from build123d import *

# Parameters (mm, degrees)
BOSS_EXTRUDE1_DEPTH = 1.905
SKETCH2_R           = 3.4925
SKETCH2_R_2         = 2.54
BOSS_EXTRUDE2_DEPTH = 50.8
FILLET2_R           = 0.635
SCALE1_SCALE        = 1.5


with BuildPart() as part:
    # Sketch1 → Boss-Extrude1 (new body)
    with BuildSketch(Plane(origin=(0, 0, 0), x_dir=(1, 0, 0), z_dir=(0, 1, 0))):
        with BuildLine():
            Line((-6.0325, -4.7625), (-6.0325, 4.7625))
            ThreePointArc((-6.0325, 4.7625), (-5.660525612, 5.660525612), (-4.7625, 6.0325))
            Line((-4.7625, 6.0325), (4.7625, 6.0325))
            ThreePointArc((4.7625, 6.0325), (5.660525612, 5.660525612), (6.0325, 4.7625))
            Line((6.0325, 4.7625), (6.0325, -4.7625))
            ThreePointArc((6.0325, -4.7625), (5.660525612, -5.660525612), (4.7625, -6.0325))
            Line((4.7625, -6.0325), (-4.7625, -6.0325))
            ThreePointArc((-4.7625, -6.0325), (-5.660525612, -5.660525612), (-6.0325, -4.7625))
        make_face()
    extrude(amount=BOSS_EXTRUDE1_DEPTH)

    # Sketch2 → Boss-Extrude2 (add)
    with BuildSketch(Plane.XZ):
        with Locations(Location((0, 0, 0), (0, 0, 270))):
            Circle(SKETCH2_R)
        with Locations(Location((0, 0, 0), (0, 0, 270))):
            Circle(SKETCH2_R_2, mode=Mode.SUBTRACT)
    extrude(amount=BOSS_EXTRUDE2_DEPTH)

    # Fillet2
    fillet2_edges = [part.edges().sort_by_distance(p)[0] for p in [
        (-5.660525612, 1.905, -5.660525612),
        (0, 0, -6.0325),
        (5.660525612, 0, -5.660525612),
        (-6.0325, 1.905, 0),
        (-5.660525612, 1.905, 5.660525612),
        (0, 1.905, 6.0325),
        (5.660525612, 1.905, 5.660525612),
        (6.0325, 1.905, 0),
        (5.660525612, 1.905, -5.660525612),
        (0, 1.905, -6.0325),
        (6.0325, 0, 0),
        (5.660525612, 0, 5.660525612),
        (0, 0, 6.0325),
        (-5.660525612, 0, 5.660525612),
        (-6.0325, 0, 0),
        (-5.660525612, 0, -5.660525612),
    ]]
    fillet(fillet2_edges, radius=FILLET2_R)


with BuildPart() as part_1:
    # Scale1: scaled about (0, -19.460130845, 0)
    add(part.part.scale(SCALE1_SCALE).moved(Location((0, 9.730065422, 0))))


solid = part_1.part
Read the model definition and answer for the solid it produces. Units are mm, in the model's axes. A direction names the side the tool comes from. Round coordinates to 2 decimals unless told otherwise and drop trailing zeros. Loops run counter-clockwise (first coordinate to the right, second up) from the corner with the lowest first, then second, coordinate; pieces in that order, holes last.
Q1. Which of the six approach directions +Z, -Z, +X, -X, +Y, -Y give full straight-line access (tool end or side, diameter ignored) to faces 1 (the face through (0, 9.73, 0)), 2 (the face through (8.506, 11.152, 8.476))?
Q2. Section A-A on z = 0 is taken. Write down the section's boundary in (x, y) (1 decimal), and give its area (3 significant figures).
Q3. Section B-B on x = -6.25 is taken. Write down the section's boundary in (y, z) (1 decimal), and give its area (3 significant figures).
Q4. Section D-D on x = 0 is taken. Write down the section's boundary in (y, z) (1 decimal).
Q5. Each of these flat-tipped pins is pushed along its axis until it touches: pin 1 (8 mm diameter, centred on y = -41, z = -4, fed in from -X); pin 2 (5 mm diameter, centred on x = 3, y = -2, fed in from +Z); pin 3 (4 mm diameter, centred on x = 2, y = -39, fed in from -Z). Where does it stop, or does it pass through?
Q6. Determine the mould class of faces 3 (the face through (-8.506, 11.152, -8.476)), 4 (the face through (0, 12.588, 0)), 5 (the face through (3.778, -27.837, 0.496)) for opening direction X: released by +X, released by -X, zero draft, split by the parting line, or undercut.
Q7. Consider probe 1 along X at (y, z) = (-26, 0); probe 2 along X at (y, z) = (3.5, 1.5); probe 3 along Z at (x, y) = (-2, -25). Determine where each line is inside the solid, lowest interval first.
Q8. Section C-C on y = -28.5 is taken. Write down the section's boundary in (x, z), and give its area (3 significant figures).
Output:
1. face 1: -Y
1. face 2: +Z, +X, +Y, -Y
2. outline: (-9, 10.7) arc R1 ccw to (-8.1, 9.7) - (-5.2, 9.7) - (-5.2, -66.5) - (-3.8, -66.5) - (-3.8, 9.7) - (3.8, 9.7) - (3.8, -66.5) - (5.2, -66.5) - (5.2, 9.7) - (8.1, 9.7) arc R1 ccw to (9, 10.7) - (9, 11.6) arc R1 ccw to (8.1, 12.6) - (-8.1, 12.6) arc R1 ccw to (-9, 11.6) - close
2. area: 269 mm2
3. outline: (9.7, -8.1) arc R1 ccw to (10.7, -9) - (11.6, -9) arc R1 ccw to (12.6, -8.1) - (12.6, 8.1) arc R1 ccw to (11.6, 9) - (10.7, 9) arc R1 ccw to (9.7, 8.1) - close
3. area: 50.9 mm2
4. outline: (-66.5, -5.2) - (9.7, -5.2) - (9.7, -8.1) arc R1 ccw to (10.7, -9) - (11.6, -9) arc R1 ccw to (12.6, -8.1) - (12.6, 8.1) arc R1 ccw to (11.6, 9) - (10.7, 9) arc R1 ccw to (9.7, 8.1) - (9.7, 5.2) - (-66.5, 5.2) - (-66.5, 3.8) - (9.7, 3.8) - (9.7, -3.8) - (-66.5, -3.8) - close
5. pin 1: stops at x = -5.24
5. pin 2: stops at z = 5.21
5. pin 3: stops at z = -5.24
6. face 3: released by -X
6. face 4: zero draft
6. face 5: undercut
7. probe 1: x = -5.24 to -3.81, 3.81 to 5.24
7. probe 2: x = -5.02 to -3.5, 3.5 to 5.02
7. probe 3: z = -4.84 to -3.24, 3.24 to 4.84
8. outline: circle Ø10.48 at (0, 0); hole circle Ø7.62 at (0, 0)
8. area: 40.6 mm2
